CAD build for the part. Positions are in the model's coordinates, mm. A direction names the side the tool comes from. Give positions to 0.01 mm unless a question says otherwise; leave off trailing zeros. Loops run counter-clockwise (first coordinate to the right, second up) from the corner with the lowest first, then second, coordinate; pieces in that order, holes last. Notation, with made-up numbers: (77, 14.25) -> (102, 14.25) arc R31 ccw to (102, 43.25) -> close; hole circle Ø9 at (9.25, -9). An arc over 180 degrees is marked (long way). Write each question's results on one line, items separated by ' | '. Start each with the question number.
```python
from build123d import *

# Parameters (mm, degrees)
SKETCH_1_W      = 30
SKETCH_1_H      = 68
SKETCH_1_R      = 1.25
EXTRUDE_6_DEPTH = 1.5
CHAMFER_2_SIZE  = 2
SKETCH_9_W      = 3.5
SKETCH_9_H      = 5
EXTRUDE_7_DEPTH = 2


with BuildPart() as part:
    # Эскиз1 → Бобышка-Вытянуть6 (new body)
    with BuildSketch(Plane.XY):
        with Locations((15, 34)):
            Rectangle(SKETCH_1_W, SKETCH_1_H)
        with Locations((15, 64)):
            Circle(SKETCH_1_R, mode=Mode.SUBTRACT)
        with Locations((4, 4)):
            Circle(SKETCH_1_R, mode=Mode.SUBTRACT)
        with Locations((26, 4)):
            Circle(SKETCH_1_R, mode=Mode.SUBTRACT)
    extrude(amount=EXTRUDE_6_DEPTH)

    # Фаска2
    chamfer_2_edges = [part.edges().sort_by_distance(p)[0] for p in [
        (0, 68, 0.75),
        (30, 68, 0.75),
        (30, 0, 0.75),
        (0, 0, 0.75),
    ]]
    chamfer(chamfer_2_edges, length=CHAMFER_2_SIZE)

    # Эскиз9 → Бобышка-Вытянуть7 (add)
    with BuildSketch(Plane.XY.offset(1.5)):
        with Locations((6.75, 63.5)):
            Rectangle(SKETCH_9_W, SKETCH_9_H)
        with Locations((23.25, 63.5)):
            Rectangle(SKETCH_9_W, SKETCH_9_H)
    extrude(amount=EXTRUDE_7_DEPTH)


solid = part.part
```
Q1. Drop flat-ended pins along their axis: pin 1 (12 mm diameter, centred on x = 11.5, y = 31, fed in from +Z); pin 2 (1.6 mm diameter, centred on y = 64, z = 2.5, fed in from +X); pin 3 (0.6 mm diameter, centred on x = 6.5, z = 3, fed in from -Y). Give the stop position or say it passes through.
Q2. Which spindle directions (+Z, -Z, +X, -X, +Y, -Y) get a long thin tool onto all of the face, cutting with end or side? Do faces 1 (the face through (7, 66, 2)), 2 (the face through (23, 61, 2)), 3 (the face through (8.5, 63, 2)). Say none if no direction does.
Q3. Mould opens along Y. For faces 4 (the face through (4.577, 2.891, 0.74)), 5 (the face through (0, 34, 1)), 6 (the face through (29, 1, 1)) say: pulls with the +Y half, pulls with the -Y half, needs draft (parallel to the pull), parting line crosses it, or undercut.
Q4. Saw through at C-C, the plane y = 4. List the corners of the cut face in (x, z), then the cut area to 3 significant figures.
Q5. Saw through at B-B, the plane z = 2.1. List the corners of the cut face in (x, y), then the cut area to 3 significant figures.
Q6. Wall check: L1, parallel to X at y = 64, z = 0.7; L2, parallel to Y at x = 26, z = 0.85; L3, parallel to Y at x = 15, z = 1.1. Give the ranges that are in metal, low to high.
Q7. Saw through at A-A, the plane x = 26. List the corners of the cut face in (y, z), then the cut area to 4 significant figures.
Q8. Saw through at D-D, the plane y = 60. List the corners of the cut face in (x, z), then the cut area to 3 significant figures.
Answer block:
1) pin 1: stops at z = 1.5 | pin 2: stops at x = 25 | pin 3: stops at y = 61
2) face 1: +Z, +X, -X, +Y | face 2: +Z, +X, -X, -Y | face 3: +Z, +Y, -Y
3) face 4: undercut | face 5: needs draft | face 6: pulls with the -Y half
4) outline: (0, 0) -> (2.75, 0) -> (2.75, 1.5) -> (0, 1.5) -> close; (5.25, 0) -> (24.75, 0) -> (24.75, 1.5) -> (5.25, 1.5) -> close; (27.25, 0) -> (30, 0) -> (30, 1.5) -> (27.25, 1.5) -> close | area: 37.5 mm2
5) outline: (5, 61) -> (8.5, 61) -> (8.5, 66) -> (5, 66) -> close; (21.5, 61) -> (25, 61) -> (25, 66) -> (21.5, 66) -> close | area: 35.0 mm2
6) L1: x = 0 to 13.75, 16.25 to 30 | L2: y = 0 to 2.75, 5.25 to 68 | L3: y = 0 to 62.75, 65.25 to 68
7) outline: (0, 0) -> (2.75, 0) -> (2.75, 1.5) -> (0, 1.5) -> close; (5.25, 0) -> (68, 0) -> (68, 1.5) -> (5.25, 1.5) -> close | area: 98.25 mm2
8) outline: (0, 0) -> (30, 0) -> (30, 1.5) -> (0, 1.5) -> close | area: 45.0 mm2
